The listing builds one solid part. Answer for the finished solid, in the listing's coordinates (mm). Coordinates: 2 decimals unless noted, no trailing zeros. Order: outer loops, then holes, each group sorted by start corner. A loop starts at its lowest first (then second) coordinate and runs counter-clockwise, first axis right, second up. Notation, with made-up numbers: (34, 2) -> (71, 2) arc R20 ccw to (71, 8) -> close; hole circle Ø5 at (51, 87). An arc over 180 degrees is marked (long way). Write each question's results on one line, items separated by ' | '. Start each with the question number.
(1) The part is cut by section A-A, the plane x = 0. Give the vertices of the cut face in (y, z).
(2) Straight lines are drawn through the part: L1, parallel to Y at x = 0, z = 11.5; L2, parallel to Z at x = 8.5, y = 3.75; L3, parallel to Y at x = -5.5, z = 7. For each, find the intervals that lie inside material, in ascending order.
(3) Given pin 1 (6.5 mm diameter, centred on x = -4, y = -2, fed in from +Z); pin 2 (6 mm diameter, centred on y = 5.5, z = 5, fed in from +X); pin 3 (8 mm diameter, centred on x = 7.5, z = 8, fed in from -Y); pin 4 (1 mm diameter, centred on x = -0.5, y = 4.5, fed in from -Z), each flat-ended and moving along its own axis, determine where each tip first touches the part or whether it passes through.
(4) The part is cut by section D-D, the plane x = -9.5. Give the vertices of the cut face in (y, z), then the cut area to 3 significant figures.
(5) The part is cut by section C-C, the plane z = 29.5. Give the vertices of the cut face in (x, y), then the cut area to 3 significant figures.
(6) Determine the mould class of faces 1 (the face through (-1.73, -7.81, 19.75)), 2 (the face through (6.466, -2.681, 18.748)), 3 (the face through (2, -9, 1)) for opening direction X: +X half, -X half, draft (parallel to the pull), parting line (faces both ways), or undercut.
```python
from build123d import *

# Parameters (mm, degrees)
F0_R     = 11
F0_R_2   = 8
F1_DEPTH = 1
F0_R_3   = 7
F2_DEPTH = 39
F3_SIZE  = 1


# Not quite as in the source:
# - a fillet or chamfer that OpenCascade refuses, or shapes differently, is made with other operations: its cross-section is extruded or revolved along the edge and cut away or added


with BuildPart() as f1:
    # F0 (on Top) → F1 (new body)
    with BuildSketch(Plane.XY):
        Circle(F0_R)
        Circle(F0_R_2, mode=Mode.SUBTRACT)
    extrude(amount=F1_DEPTH)

    # F0 (on Top) → F2 (join)
    with BuildSketch(Plane.XY):
        Circle(F0_R_2)
        Circle(F0_R_3, mode=Mode.SUBTRACT)
    extrude(amount=F2_DEPTH)

    # F3
    f3_edges = [f1.edges().sort_by_distance(p)[0] for p in [
        (-8, 0, 1),
        (-7, 0, 0),
    ]]
    chamfer(f3_edges, length=F3_SIZE)

    # F4: chamfer of 2 on 1 edges, made by hand

    # F4_s1 → F4_t2 (revolve, cut)
    with BuildSketch(Plane.XZ):
        Polygon((7, 37), (9, 39), (7, 39), align=None)
    revolve(axis=Axis((0, 0, 39), (0, 0, 1)), mode=Mode.SUBTRACT)


solid = f1.part
```
Established:
1) outline: (-11, 0) -> (-8, 0) -> (-7, 1) -> (-7, 37) -> (-8, 38) -> (-8, 2) -> (-9, 1) -> (-11, 1) -> close; (7, 1) -> (8, 0) -> (11, 0) -> (11, 1) -> (9, 1) -> (8, 2) -> (8, 38) -> (7, 37) -> close
2) L1: y = -8 to -7, 7 to 8 | L2: z = 0 to 1 | L3: y = -5.81 to -4.33, 4.33 to 5.81
3) pin 1: stops at z = 37.72 | pin 2: stops at x = 7.6 | pin 3: stops at y = -7.19 | pin 4: passes through
4) outline: (-5.55, 0) -> (5.55, 0) -> (5.55, 1) -> (-5.55, 1) -> close | area: 11.1 mm^2
5) outline: circle Ø16 at (0, 0); hole circle Ø14 at (0, 0) | area: 47.1 mm^2
6) face 1: parting line | face 2: undercut | face 3: draft
